from build123d import *

# Parameters (mm, degrees)
F0_W     = 253.456043
F0_H     = 76.289
F1_DEPTH = 139.7
F0_W_2   = 356.663674
F0_H_2   = 128.946438
F2_DEPTH = 19.05


with BuildPart() as f1:
    # F0 (on Top) → F1 (new body)
    with BuildSketch(Plane.XY):
        with Locations((156.799115, -68.734861)):
            Rectangle(F0_W, F0_H)
    extrude(amount=F1_DEPTH)

    # F0 (on Top) → F2 (join)
    with BuildSketch(Plane.XY):
        with Locations((178.331837, -64.473219)):
            Rectangle(F0_W_2, F0_H_2)
        with Locations((156.799115, -68.734861)):
            Rectangle(F0_W, F0_H, mode=Mode.SUBTRACT)
    extrude(amount=F2_DEPTH)


solid = f1.part
Verification items for the finished model (mm, model axes). A direction names the side the tool comes from. Give positions to 0.01 mm unless a question says otherwise; leave off trailing zeros. Order: outer loops, then holes, each group sorted by start corner. A loop starts at its lowest first (then second) coordinate and runs counter-clockwise, first axis right, second up. Notation, with made-up numbers: M 83.25,52 L 139.25,52 A20 cw 139.25,89 Z; hole C 11,49 d2. An arc over 180 degrees is marked long. Answer as a JSON object with one key per item and string values. Group by question number.
1) Cross-section at C-C (z = 103). Enter the section's corners in (x, y).
2) Depth check by flat-ended pin: pin 1 Ø3 at (y, z) = (-60.5, 70) entering from -X; pin 2 Ø2 at (x, z) = (209, 102.5) entering from +Y; pin 3 Ø1 at (y, z) = (-57, 62) entering from +X. Enter the tip coordinate at first touch or a pass-through.
3) Cross-section at D-D (x = 327.5). Enter the section's corners in (y, z).
4) Scan lines: line 1 along Y through (x, z) = (131.5, 36); line 2 along Z through (x, y) = (29, -78.5); line 3 along X through (y, z) = (-51, 42). Record each from-to range of solid material in increasing order. Write a range as [from, to].
5) Cross-section at A-A (x = 52.5). Enter the section's corners in (y, z).
6) Access from +Z, -Z, +X, -X, +Y, -Y to the whole of each face (thin tool, end or side, straight path). Record for faces 1 (the face through (155, -30.59, 79)), 2 (the face through (155, -106.879, 79)), 3 (the face through (283.527, -69, 79)).
7) Cross-section at B-B (y = -99). Enter the section's corners in (x, z), then the cut area to 3 significant figures.
Result sheet:
{
 "1": {"outline": "M 30.07,-106.88 L 283.53,-106.88 L 283.53,-30.59 L 30.07,-30.59 Z"},
 "2": {"pin 1": "stops at x = 30.07", "pin 2": "stops at y = -30.59", "pin 3": "stops at x = 283.53"},
 "3": {"outline": "M -128.95,0 L 0,0 L 0,19.05 L -128.95,19.05 Z"},
 "4": {"line 1": "y = [-106.88, -30.59]", "line 2": "z = [0, 19.05]", "line 3": "x = [30.07, 283.53]"},
 "5": {"outline": "M -128.95,0 L 0,0 L 0,19.05 L -30.59,19.05 L -30.59,139.7 L -106.88,139.7 L -106.88,19.05 L -128.95,19.05 Z"},
 "6": {"face 1": "+Z, +X, -X, +Y", "face 2": "+Z, +X, -X, -Y", "face 3": "+Z, +X, +Y, -Y"},
 "7": {"outline": "M 0,0 L 356.66,0 L 356.66,19.05 L 283.53,19.05 L 283.53,139.7 L 30.07,139.7 L 30.07,19.05 L 0,19.05 Z", "area": "37,400 mm2"}
}
